Design review of the part built by this model. Coordinates are the model's own, in mm. A direction names the side the tool comes from. Round coordinates to 2 decimals unless told otherwise and drop trailing zeros. Order: outer loops, then holes, each group sorted by start corner. A loop starts at its lowest first (then second) coordinate and runs counter-clockwise, first axis right, second up. Notation, with made-up numbers: (11.5, 78) - (66.5, 78) arc R9 cw to (66.5, 83) - close; hole circle Ø8 at (18, -23.75). An arc over 180 degrees is marked (long way). Write item = value, one per line.
from build123d import *

# Parameters (mm, degrees)
BOSS_EXTRUDE1_DEPTH = 12
BOSS_EXTRUDE2_DEPTH = 5
CUT_EXTRUDE1_START  = -19
CUT_EXTRUDE1_DEPTH  = 29
SKETCH4_R           = 2
BOSS_EXTRUDE3_DEPTH = 3
FILLET1_R           = 0.5


with BuildPart() as part:
    # Sketch1 → Boss-Extrude1 (new body)
    with BuildSketch(Plane.XY):
        Polygon((11, 7), (16, 7), (16, 5), (11, 5), (11, -11), (-11, -11), (-11, 5), (-16, 5), (-16, 7), (-11, 7), (-11, 11), (11, 11), align=None)
    extrude(amount=-BOSS_EXTRUDE1_DEPTH)

    # Sketch2 → Boss-Extrude2 (add)
    with BuildSketch(Plane(origin=(0, 11, 0), x_dir=(1, 0, 0), z_dir=(0, 1, 0))):
        with BuildLine():
            Line((1.499090834, 8.4), (0.499090834, 8.4))
            ThreePointArc((0.499090834, 8.4), (-11, 6), (0.499090834, 3.6))
            Line((0.499090834, 3.6), (1.499090834, 3.6))
            ThreePointArc((1.499090834, 3.6), (3.899090834, 6), (1.499090834, 8.4))
        make_face()
    extrude(amount=BOSS_EXTRUDE2_DEPTH)

    # Sketch3 → Cut-Extrude1 (cut)
    with BuildSketch(Plane(origin=(0, 7, 0), x_dir=(1, 0, 0), z_dir=(0, 1, 0)).offset(CUT_EXTRUDE1_START)):
        with BuildLine():
            Line((15.2, 6.5), (16, 6.5))
            Line((16, 6.5), (16, 5.5))
            Line((16, 5.5), (15.2, 5.5))
            ThreePointArc((15.2, 5.5), (12.285786438, 6), (15.2, 6.5))
        make_face()
    cut_extrude1 = extrude(amount=CUT_EXTRUDE1_DEPTH, mode=Mode.SUBTRACT)

    # Mirror1: Cut-Extrude1 across plane
    add(cut_extrude1.mirror(Plane(origin=(0, 0, 0), x_dir=(0, 0, 1), z_dir=(1, 0, 0))), mode=Mode.SUBTRACT)

    # Sketch4 → Boss-Extrude3 (add)
    with BuildSketch(Plane(origin=(0, 16, 0), x_dir=(1, 0, 0), z_dir=(0, 1, 0))):
        with Locations((-5, 6)):
            Circle(SKETCH4_R)
    extrude(amount=BOSS_EXTRUDE3_DEPTH)

    # Fillet1
    fillet1_edges = [part.edges().sort_by_distance(p)[0] for p in [
        (0.499090834, 13.5, -8.4),
        (0.499090834, 13.5, -3.6),
    ]]
    fillet(fillet1_edges, radius=FILLET1_R)


solid = part.part
Item 1: For faces 4 (the face through (-12.9, 5, -4.6)), 5 (the face through (6, 11, -6)), 6 (the face through (11, 9, -6)), list the 3-axis set-ups (+Z, -Z, +X, -X, +Y, -Y) from which the entire face can be reached by the end or side of a thin tool; tool diameter is ignored.
Data:
face_4 = +Z, -Z, -X, -Y
face_5 = +X, +Y
face_6 = +Z, -Z, +X, +Y
Item 2: Take a section at A-A, the plane z = -7. State the section outline as (x, y) points.
Data:
outline = (-16, 5) - (-14.9, 5) - (-14.9, 7) - (-16, 7) - close; (-12.67, 5) - (-11, 5) - (-11, -11) - (11, -11) - (11, 5) - (12.67, 5) - (12.67, 7) - (11, 7) - (11, 11) - (3.68, 11) - (3.68, 16) - (-3.27, 16) - (-3.27, 19) - (-6.73, 19) - (-6.73, 16) - (-10.92, 16) - (-10.92, 11) - (-11, 11) - (-11, 7) - (-12.67, 7) - close; (14.9, 5) - (16, 5) - (16, 7) - (14.9, 7) - close
Item 3: Take a section at B-B, the plane y = 6. State the section outline as (x, z) points, and give its area (3 significant figures).
Data:
outline = (-16, -12) - (16, -12) - (16, -6.5) - (15.2, -6.5) arc R1.5 cw (long way) to (15.2, -5.5) - (16, -5.5) - (16, 0) - (-16, 0) - (-16, -5.5) - (-15.2, -5.5) arc R1.5 cw (long way) to (-15.2, -6.5) - (-16, -6.5) - close
area = 368 mm2
Item 4: The part is to be moulded in two halves that separate along Z. For faces 1 (the face through (-16, 6, -3)), 2 (the face through (-6.474, 17.479, -7.352)), 3 (the face through (15.6, 6, -6.5)), say which applies: +Z half, -Z half, draft (parallel to the pull), parting line (faces both ways), or undercut.
Data:
face_1 = draft
face_2 = parting line
face_3 = undercut
Item 5: For line 1 along X through (y, z) = (5.9, -6); line 2 along X through (y, z) = (7.5, -7); line 3 along Y through (x, z) = (-2, -7), list the stretches that pass through material, from the lowest coordinate up. Write a range as [from, to].
Data:
line_1 = [-12.29, 12.29]
line_2 = [-11, 11]
line_3 = [-11, 16]
Item 6: Insertion check: P1, Ø1.2, axis at y = 8.5, z = -4.5, coming from the +X side; P2, Ø1.5, axis at x = 12.5, z = -5.5, coming from the +Y side; P3, Ø5, axis at x = 2.5, y = 0.5, coming from the +Z side; P4, Ø1.2, axis at y = 8, z = -7.5, coming from the -X side. Each pin has a flat end and moves straight along its axis. Give the tip position at first contact, or say it passes through.
Data:
P1 = 11
P2 = 7
P3 = 0
P4 = -11
Item 7: Take a section at C-C, the plane x = -14. State the section outline as (y, z) points, and give its area (3 significant figures).
Data:
outline = (5, -12) - (7, -12) - (7, -7.48) - (5, -7.48) - close; (5, -4.52) - (7, -4.52) - (7, 0) - (5, 0) - close
area = 18.1 mm2
Item 8: Take a section at D-D, the plane z = -10.5. State the section outline as (x, y) points, and give its area (3 significant figures).
Data:
outline = (-16, 5) - (-11, 5) - (-11, -11) - (11, -11) - (11, 5) - (16, 5) - (16, 7) - (11, 7) - (11, 11) - (-1.03, 11) - (-1.03, 16) - (-8.97, 16) - (-8.97, 11) - (-11, 11) - (-11, 7) - (-16, 7) - close
area = 544 mm2
